from build123d import *

# Parameters (mm, degrees)
SKETCH_1_W          = 220
SKETCH_1_H          = 180
EXTRUDE_1_DEPTH     = 4
SKETCH_2_W          = 80
SKETCH_2_H          = 80
CUT_EXTRUDE_1_DEPTH = 4
SKETCH_3_R          = 1.75
CUT_EXTRUDE_2_DEPTH = 4
SKETCH_5_R          = 1.75
CUT_EXTRUDE_3_DEPTH = 4
SKETCH_6_R          = 1.75
CUT_EXTRUDE_4_DEPTH = 4
FILLET_1_R          = 4
FILLET_2_R          = 4


with BuildPart() as part:
    # 草图1 → 凸台-拉伸1 (new body)
    with BuildSketch(Plane(origin=(0, 0, 0), x_dir=(1, 0, 0), z_dir=(0, 1, 0))):
        Rectangle(SKETCH_1_W, SKETCH_1_H)
    extrude(amount=EXTRUDE_1_DEPTH)

    # 草图2 → 切除-拉伸1 (cut)
    with BuildSketch(Plane(origin=(0, 4, 0), x_dir=(1, 0, 0), z_dir=(0, 1, 0))):
        Rectangle(SKETCH_2_W, SKETCH_2_H)
    extrude(amount=-CUT_EXTRUDE_1_DEPTH, mode=Mode.SUBTRACT)

    # 草图3 → 切除-拉伸2 (cut)
    with BuildSketch(Plane(origin=(0, 0, 0), x_dir=(-1, 0, 0), z_dir=(0, -1, 0))):
        with BuildLine():
            ThreePointArc((90.584745347, 69.545196968), (99.777133502, 73.352808813), (103.584745347, 82.545196968))
            ThreePointArc((103.584745347, 82.545196968), (105.584745347, 84.545196968), (107.584745347, 82.545196968))
            ThreePointArc((107.584745347, 82.545196968), (102.605560627, 70.524381688), (90.584745347, 65.545196968))
            ThreePointArc((90.584745347, 65.545196968), (88.584745347, 67.545196968), (90.584745347, 69.545196968))
        make_face()
        with Locations(Location((90.584745347, 82.545196968, 0), (0, 0, 90))):
            Circle(SKETCH_3_R)
        with BuildLine():
            ThreePointArc((-90.584745347, -69.545196968), (-99.777133502, -73.352808813), (-103.584745347, -82.545196968))
            ThreePointArc((-103.584745347, -82.545196968), (-105.584745347, -84.545196968), (-107.584745347, -82.545196968))
            ThreePointArc((-107.584745347, -82.545196968), (-102.605560627, -70.524381688), (-90.584745347, -65.545196968))
            ThreePointArc((-90.584745347, -65.545196968), (-88.584745347, -67.545196968), (-90.584745347, -69.545196968))
        make_face()
        with Locations(Location((-90.584745347, -82.545196968, 0), (0, 0, 90))):
            Circle(SKETCH_3_R)
        with BuildLine():
            ThreePointArc((-90.584745347, 65.545196968), (-102.605560627, 70.524381688), (-107.584745347, 82.545196968))
            ThreePointArc((-107.584745347, 82.545196968), (-105.584745347, 84.545196968), (-103.584745347, 82.545196968))
            ThreePointArc((-103.584745347, 82.545196968), (-99.777133502, 73.352808813), (-90.584745347, 69.545196968))
            ThreePointArc((-90.584745347, 69.545196968), (-88.584745347, 67.545196968), (-90.584745347, 65.545196968))
        make_face()
        with Locations(Location((-90.584745347, 82.545196968, 0), (0, 0, 90))):
            Circle(SKETCH_3_R)
        with BuildLine():
            ThreePointArc((90.584745347, -69.545196968), (99.777133502, -73.352808813), (103.584745347, -82.545196968))
            ThreePointArc((103.584745347, -82.545196968), (105.584745347, -84.545196968), (107.584745347, -82.545196968))
            ThreePointArc((107.584745347, -82.545196968), (102.605560627, -70.524381688), (90.584745347, -65.545196968))
            ThreePointArc((90.584745347, -65.545196968), (88.584745347, -67.545196968), (90.584745347, -69.545196968))
        make_face()
        with Locations(Location((90.584745347, -82.545196968, 0), (0, 0, 90))):
            Circle(SKETCH_3_R)
    extrude(amount=-CUT_EXTRUDE_2_DEPTH, mode=Mode.SUBTRACT)

    # 草图5 → 切除-拉伸3 (cut)
    with BuildSketch(Plane.XZ):
        with Locations(Location((45.401224127, 38.626328315, 0), (0, 0, 270))):
            Circle(SKETCH_5_R)
        with Locations(Location((88.581224127, 14.496328315, 0), (0, 0, 270))):
            Circle(SKETCH_5_R)
        with Locations(Location((45.401224127, -36.303671685, 0), (0, 0, 270))):
            Circle(SKETCH_5_R)
    extrude(amount=-CUT_EXTRUDE_3_DEPTH, mode=Mode.SUBTRACT)

    # 草图6 → 切除-拉伸4 (cut)
    with BuildSketch(Plane.XZ):
        with Locations(Location((-40, -80, 0), (0, 0, 270))):
            Circle(SKETCH_6_R)
        with Locations(Location((-100, -30, 0), (0, 0, 270))):
            Circle(SKETCH_6_R)
        with Locations(Location((40, -80, 0), (0, 0, 90))):
            Circle(SKETCH_6_R)
        with Locations(Location((100, -30, 0), (0, 0, 90))):
            Circle(SKETCH_6_R)
        with Locations(Location((100, 30, 0), (0, 0, 270))):
            Circle(SKETCH_6_R)
        with Locations(Location((40, 80, 0), (0, 0, 270))):
            Circle(SKETCH_6_R)
        with Locations(Location((-40, 80, 0), (0, 0, 90))):
            Circle(SKETCH_6_R)
        with Locations(Location((-100, 30, 0), (0, 0, 90))):
            Circle(SKETCH_6_R)
    extrude(amount=-CUT_EXTRUDE_4_DEPTH, mode=Mode.SUBTRACT)

    # 圆角1
    fillet_1_edges = [part.edges().sort_by_distance(p)[0] for p in [
        (110, 2, 90),
        (-110, 2, 90),
        (-110, 2, -90),
        (110, 2, -90),
    ]]
    fillet(fillet_1_edges, radius=FILLET_1_R)

    # 圆角2
    fillet_2_edges = [part.edges().sort_by_distance(p)[0] for p in [
        (-40, 2, -40),
        (40, 2, -40),
        (40, 2, 40),
        (-40, 2, 40),
    ]]
    fillet(fillet_2_edges, radius=FILLET_2_R)


solid = part.part
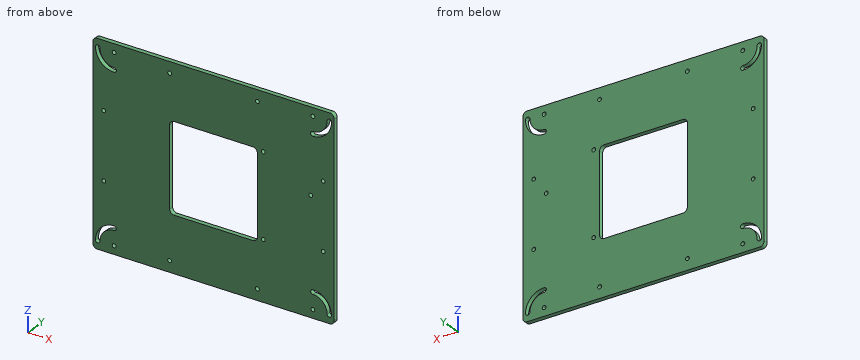
Verification items for the finished model (mm, model axes). Give positions to 0.01 mm unless a question says otherwise; leave off trailing zeros. Loops run counter-clockwise (first coordinate to the right, second up) from the corner with the lowest first, then second, coordinate; pieces in that order, holes last. Notation, with made-up numbers: (67.25, 56) - (85.25, 56) arc R14 cw to (85.25, 62) - close; hole circle Ø3 at (18, 54.5). An arc over 180 degrees is marked (long way). Write each question's results on one line, items separated by ' | '.
1) Sectioned sample at A-A on x = 1. Record the boundary of the cut face in (y, z).
Solution:
outline: (0, -90) - (4, -90) - (4, -40) - (0, -40) - close; (0, 40) - (4, 40) - (4, 90) - (0, 90) - close
2) Depth check by flat-ended pin: P1, Ø3, axis at x = 40, z = 80, coming from the -Y side. Enter the tip coordinate at first touch or a pass-through.
Solution:
P1: through
3) Material ranges on L1, parallel to Z at x = -90.5, y = 1.8; L2, parallel to Z at x = 17, y = 0.45; L3, parallel to X at y = 1.8, z = 27, recorded low to high. Write a range as from..to.
Solution:
L1: -90..-84.29, -80.8..-69.54, -65.55..65.55, 69.54..80.8, 84.29..90 | L2: -90..-40, 40..90 | L3: -110..-40, 40..110
4) Sectioned sample at B-B on y = 3. Count the separate pieces of the cut face and the enclosed holes in it, plus the area to 3 significant figures.
Solution:
separate pieces: 1 | enclosed holes: 20 | area: 32,600 mm2
